from build123d import *

# Parameters (mm, degrees)
CUT_EXTRUDE_START        = 5.5
CUT_EXTRUDE_1_DEPTH      = 146.165191733
HOLE_WIZARD_M12_1_D      = 10.2
HOLE_WIZARD_M12_1_DEPTH  = 60
HOLE_WIZARD_M12_1_TIP    = 3.064389157
CUT_EXTRUDE_2_DEPTH      = 151.665191733
CUT_EXTRUDE_2_DEPTH_BACK = 151.665191733


# Read off the part's stored shape, not the designer's step: M10 机械螺纹 螺柱1
with BuildPart() as part:
    # 草图1 → 旋转1 (revolve)
    with BuildSketch(Plane.XY, mode=Mode.PRIVATE) as revolve_1_sk:
        Polygon((0, 0), (0, 10), (4, 10), (4, 8), (130, 8), (130, 4), (133, 4), (133, 5), (150, 5), (150, 0), align=None)
    revolve(revolve_1_sk.sketch.rotate(Axis((0, 0, 0), (1, 0, 0)), 90), axis=Axis((0, 0, 0), (1, 0, 0)))

    # M10 机械螺纹 螺柱1 outline → M10 机械螺纹 螺柱1 (revolve, cut)
    with BuildSketch(Plane.YX):
        Polygon((5, 150), (4.188, 150), (5, 149.188), align=None)
    revolve(axis=Axis((0, 0, 0), (1, 0, 0)), mode=Mode.SUBTRACT)

    # 草图3 → 切除-拉伸1 (cut, through all)
    with BuildSketch(Plane(origin=(0, 0, 0), x_dir=(1, 0, 0), z_dir=(0, 1, 0)).offset(CUT_EXTRUDE_START)):
        with BuildLine():
            Line((130, -2.5), (72.5, -2.5))
            ThreePointArc((72.5, -2.5), (70, 0), (72.5, 2.5))
            Line((72.5, 2.5), (130, 2.5))
            ThreePointArc((130, 2.5), (132.5, 0), (130, -2.5))
        make_face()
    extrude(amount=CUT_EXTRUDE_1_DEPTH, mode=Mode.SUBTRACT)

    # M12 螺纹孔1
    with Locations(Plane.ZY):
        with Locations((0, 0)):
            Hole(HOLE_WIZARD_M12_1_D / 2, depth=HOLE_WIZARD_M12_1_DEPTH)
            with Locations((0, 0, -(HOLE_WIZARD_M12_1_DEPTH + HOLE_WIZARD_M12_1_TIP / 2))):  # 118° drill point
                Cone(0, HOLE_WIZARD_M12_1_D / 2, HOLE_WIZARD_M12_1_TIP, mode=Mode.SUBTRACT)

    # 草图6 → 切除-拉伸2 (cut, two sides: drawn at the far end of the back side and taken through both)
    with BuildSketch(Plane.XY.offset(-CUT_EXTRUDE_2_DEPTH_BACK)):
        Polygon((-78.518127086, -168.518127086), (82, -8), (87, -3), (102, -3), (107, -8), (267.518127086, -168.518127086), (267.518127086, -622.531951751), (-78.518127086, -622.531951751), align=None)
    extrude(amount=CUT_EXTRUDE_2_DEPTH + CUT_EXTRUDE_2_DEPTH_BACK, mode=Mode.SUBTRACT)


solid = part.part
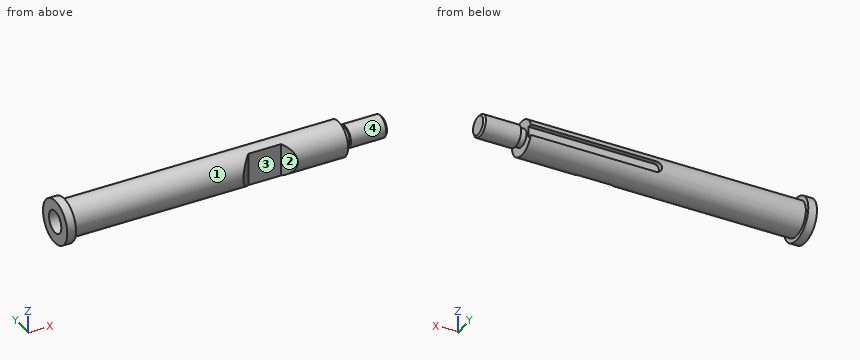
Source: CAD feature listing. Evaluate the final solid. Frame: model axes, mm. Face numbers are marked on the shaded views. A direction names the side the tool comes from. Round coordinates to 2 decimals unless told otherwise and drop trailing zeros. Loops run counter-clockwise (first coordinate to the right, second up) from the corner with the lowest first, then second, coordinate; pieces in that order, holes last.
Q1. Section B-B, the plane x = 50.5. Return loops of the section in (y, z), plus the area to 3 significant figures.
Q2. Section D-D, the plane x = 127. Return loops of the section in (y, z).
Q3. Section C-C, the plane x = 67. Return loops of the section in (y, z).
Q4. Section A-A, the plane x = 93. Return loops of the section in (y, z), plus the area to 3 significant figures.
Q5. First-contact query: P1, Ø0.6, axis at x = 102, y = 6, coming from the +Z side; P2, Ø1, axis at y = 2, z = -3, coming from the -X side; P3, Ø5, axis at x = 87.5, y = -0.5, coming from the +Z side. Flat tips, straight axial feed; report the tip coordinate or a pass-through.
Q6. Mould query, pull axis X, two halves, no side actions, for the marked faces 3 and 4. Classes: pulls with the +X half, pulls with the -X half, needs draft (parallel to the pull), parting line crosses it, or undercut.
Q7. Ray query, line 1 (Y direction, x = 39, z = 0); line 2 (X direction, y = 1.5, z = 8.25); line 3 (Y direction, x = 30, z = 4). Return the intervals inside material, ascending.
Q8. Access query for the marked faces 1 and 2. Directions: +Z, -Z, +X, -X, +Y, -Y. A direction counts if a zero-diameter tool reaches every point of the face in a straight line with its end or side. Return the directions, or none.
Solutions:
1. outline: circle Ø16 at (0, 0); hole circle Ø10.2 at (0, 0)
1. area: 119 mm2
2. outline: (5.5, -2.5) - (5.5, 2.5) - (7.6, 2.5) arc R8 ccw (long way) to (7.6, -2.5) - close
3. outline: circle Ø16 at (0, 0)
4. outline: (-3, -7.42) arc R8 ccw to (7.6, -2.5) - (5.5, -2.5) - (5.5, 2.5) - (7.6, 2.5) arc R8 ccw to (-3, 7.42) - close
4. area: 136 mm2
5. P1: stops at z = 5.61
5. P2: stops at x = 60.6
5. P3: stops at z = 8
6. face 3: undercut
6. face 4: needs draft
7. line 1: y = -8 to -5.1, 5.1 to 8
7. line 2: x = 0 to 4
7. line 3: y = -6.93 to -3.16, 3.16 to 6.93
8. face 1: +X
8. face 2: +Z, -Z, -Y
